from build123d import *

# Parameters (mm, degrees)
SKETCH1_W           = 28.4988
SKETCH1_H           = 51.943
SKETCH1_R           = 1.4986
BOSS_EXTRUDE1_DEPTH = 1.6002
SKETCH2_W           = 2.54
SKETCH2_H           = 38.1
BOSS_EXTRUDE2_DEPTH = 8.2042
SKETCH3_W           = 15.748
SKETCH3_H           = 17.78
BOSS_EXTRUDE3_DEPTH = 3.2258
SKETCH4_W           = 40.132
SKETCH4_H           = 60.198
SKETCH4_R           = 1.0795
BOSS_EXTRUDE4_DEPTH = 1.6002


with BuildPart() as part:
    # Sketch1 → Boss-Extrude1 (new body)
    with BuildSketch(Plane(origin=(0, 0, 0), x_dir=(1, 0, 0), z_dir=(0, 1, 0))):
        Rectangle(SKETCH1_W, SKETCH1_H)
        with Locations((-11.7602, 23.3299)):
            Circle(SKETCH1_R, mode=Mode.SUBTRACT)
        with Locations((11.7602, -23.3299)):
            Circle(SKETCH1_R, mode=Mode.SUBTRACT)
        with Locations((-11.7602, -23.3299)):
            Circle(SKETCH1_R, mode=Mode.SUBTRACT)
        with Locations((11.7602, 23.3299)):
            Circle(SKETCH1_R, mode=Mode.SUBTRACT)
    extrude(amount=BOSS_EXTRUDE1_DEPTH)

    # Sketch2 → Boss-Extrude2 (add)
    with BuildSketch(Plane(origin=(0, 1.6002, 0), x_dir=(1, 0, 0), z_dir=(0, 1, 0))):
        with Locations((-12.9794, 0)):
            Rectangle(SKETCH2_W, SKETCH2_H)
        with Locations((12.9794, 0)):
            Rectangle(SKETCH2_W, SKETCH2_H)
    extrude(amount=BOSS_EXTRUDE2_DEPTH)

    # Sketch3 → Boss-Extrude3 (add)
    with BuildSketch(Plane.XZ):
        with Locations((0, 9.4615)):
            Rectangle(SKETCH3_W, SKETCH3_H)
    extrude(amount=BOSS_EXTRUDE3_DEPTH)

    # Sketch4 → Boss-Extrude4 (add)
    with BuildSketch(Plane(origin=(0, 5.6134, 0), x_dir=(1, 0, 0), z_dir=(0, 1, 0))):
        with Locations((-1.756423699, 3.175)):
            Rectangle(SKETCH4_W, SKETCH4_H)
        with Locations((-18.710923699, 30.0355)):
            Circle(SKETCH4_R, mode=Mode.SUBTRACT)
        with Locations((15.198076301, 30.0355)):
            Circle(SKETCH4_R, mode=Mode.SUBTRACT)
        with Locations((15.198076301, -23.6855)):
            Circle(SKETCH4_R, mode=Mode.SUBTRACT)
        with Locations((-18.710923699, -23.6855)):
            Circle(SKETCH4_R, mode=Mode.SUBTRACT)
    extrude(amount=BOSS_EXTRUDE4_DEPTH)


solid = part.part
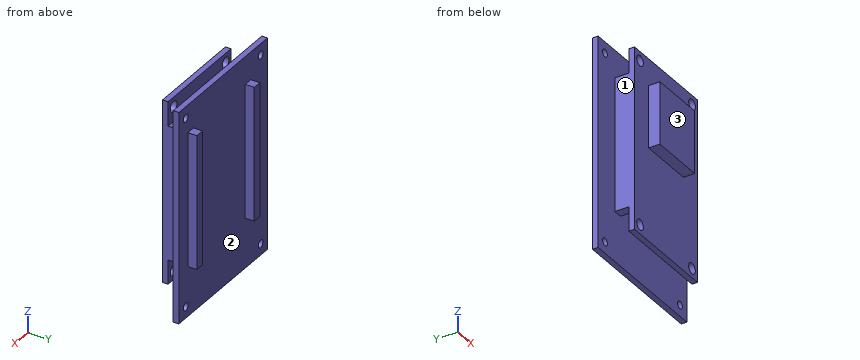
Can you work these out from the model? Positions are in its coordinate system, mm. Face numbers are marked on the shaded views. Give positions to 0.01 mm unless a question says otherwise; leave off trailing zeros. Loops run counter-clockwise (first coordinate to the right, second up) from the corner with the lowest first, then second, coordinate; pieces in that order, holes last. Notation, with made-up numbers: (88.5, -9.75) - (139.5, -9.75) arc R21 cw to (139.5, 11.25) - close; hole circle Ø10 at (15, -23.5). An arc over 180 degrees is marked (long way). One line per item, written item: value.
(1) If we section it at B-B, the plane z = 20.5: List the corners of the cut face in (x, y) for me, plus the area to 3 significant figures.
Verdict:
outline: (-21.82, 5.61) - (18.31, 5.61) - (18.31, 7.21) - (-21.82, 7.21) - close; (-14.25, 0) - (14.25, 0) - (14.25, 1.6) - (-14.25, 1.6) - close
area: 110 mm^2
(2) If we mould it in two halves opening along X, with no side actions, what happens to the marked faces 1, 2 and 3? For each: released by +X, released by -X, zero draft, split by the parting line, or undercut.
Verdict:
face 1: released by -X
face 2: undercut
face 3: zero draft
(3) If we section it at C-C, the plane x = -1: List the corners of the cut face in (y, z) for me.
Verdict:
outline: (-3.23, 0.57) - (0, 0.57) - (0, -25.97) - (1.6, -25.97) - (1.6, 25.97) - (0, 25.97) - (0, 18.35) - (-3.23, 18.35) - close; (5.61, -33.27) - (7.21, -33.27) - (7.21, 26.92) - (5.61, 26.92) - close
(4) If we section it at A-A, the plane y = 4.25: List the corners of the cut face in (x, z) for me, plus the area to 3 significant figures.
Verdict:
outline: (-14.25, -19.05) - (-11.71, -19.05) - (-11.71, 19.05) - (-14.25, 19.05) - close; (11.71, -19.05) - (14.25, -19.05) - (14.25, 19.05) - (11.71, 19.05) - close
area: 194 mm^2
(5) I need wall thicknesses on line 1 along Y through (x, z) = (2, 15); line 2 along Y through (x, z) = (12, -20.5); line 3 along X through (y, z) = (7.5, 15). Which ranges of each line are inside material? Lowest first, please.
Verdict:
line 1: -3.23 to 1.6, 5.61 to 7.21
line 2: 0 to 1.6, 5.61 to 7.21
line 3: -14.25 to -11.71, 11.71 to 14.25
(6) I'm going to push flat-ended pins straight in: pin 1 (1.5 mm diameter, centred on x = 11, z = 5, fed in from +Y); pin 2 (10 mm diameter, centred on x = -15, z = 16, fed in from -Y); pin 3 (1.3 mm diameter, centred on y = 8, z = -8.5, fed in from -X); pin 4 (2 mm diameter, centred on x = 13, y = 8.5, fed in from -Z). Where does each tip first touch, or does it pass through?
Verdict:
pin 1: y = 9.8
pin 2: y = 0
pin 3: x = -14.25
pin 4: z = -19.05
(7) If we section it at D-D, the plane z = -6: List the corners of the cut face in (x, y) for me, plus the area to 3 significant figures.
Verdict:
outline: (-21.82, 5.61) - (-14.25, 5.61) - (-14.25, 0) - (14.25, 0) - (14.25, 5.61) - (18.31, 5.61) - (18.31, 7.21) - (14.25, 7.21) - (14.25, 9.8) - (11.71, 9.8) - (11.71, 7.21) - (-11.71, 7.21) - (-11.71, 9.8) - (-14.25, 9.8) - (-14.25, 7.21) - (-21.82, 7.21) - close; hole (-11.71, 1.6) - (11.71, 1.6) - (11.71, 5.61) - (-11.71, 5.61) - close
area: 143 mm^2
